```python
from build123d import *

# Parameters (mm, degrees)
SKETCH1_W           = 740
SKETCH1_H           = 720
SKETCH1_W_2         = 720
SKETCH1_H_2         = 700
BOSS_EXTRUDE1_DEPTH = 15
SKETCH2_R           = 2.5
CUT_EXTRUDE1_DEPTH  = 517.454257413
SKETCH3_W           = 20
SKETCH3_H           = 10
CUT_EXTRUDE2_DEPTH  = 20
SKETCH5_W           = 20
SKETCH5_H           = 10
CUT_EXTRUDE3_DEPTH  = 20
SKETCH6_W           = 20
SKETCH6_H           = 30
SKETCH6_W_2         = 30
SKETCH6_H_2         = 20
BOSS_EXTRUDE2_DEPTH = 4
SKETCH7_R           = 2
CUT_EXTRUDE4_DEPTH  = 4


with BuildPart() as part:
    # Sketch1 → Boss-Extrude1 (new body)
    with BuildSketch(Plane(origin=(0, 0, 0), x_dir=(1, 0, 0), z_dir=(0, 1, 0))):
        Rectangle(SKETCH1_W, SKETCH1_H)
        Rectangle(SKETCH1_W_2, SKETCH1_H_2, mode=Mode.SUBTRACT)
    extrude(amount=BOSS_EXTRUDE1_DEPTH)

    # Sketch2 → Cut-Extrude1 (cut, through all)
    with BuildSketch(Plane(origin=(0, 15, 0), x_dir=(1, 0, 0), z_dir=(0, 1, 0))):
        with Locations(Location((-365, 355, 0), (0, 0, 270))):
            Circle(SKETCH2_R)
        with Locations(Location((365, 355, 0), (0, 0, 270))):
            Circle(SKETCH2_R)
        with Locations(Location((365, -355, 0), (0, 0, 270))):
            Circle(SKETCH2_R)
        with Locations(Location((-365, -355, 0), (0, 0, 270))):
            Circle(SKETCH2_R)
    extrude(amount=-CUT_EXTRUDE1_DEPTH, mode=Mode.SUBTRACT)

    # Sketch3 → Cut-Extrude2 (cut)
    with BuildSketch(Plane.XY.offset(360)):
        with Locations((-360, 7.5)):
            Rectangle(SKETCH3_W, SKETCH3_H)
        with Locations((360, 7.5)):
            Rectangle(SKETCH3_W, SKETCH3_H)
    extrude(amount=-CUT_EXTRUDE2_DEPTH, mode=Mode.SUBTRACT)

    # Sketch5 → Cut-Extrude3 (cut)
    with BuildSketch(Plane(origin=(0, 0, -360), x_dir=(-1, 0, 0), z_dir=(0, 0, -1))):
        with Locations((-360, 7.5)):
            Rectangle(SKETCH5_W, SKETCH5_H)
        with Locations((360, 7.5)):
            Rectangle(SKETCH5_W, SKETCH5_H)
    extrude(amount=-CUT_EXTRUDE3_DEPTH, mode=Mode.SUBTRACT)

    # Sketch6 → Boss-Extrude2 (add)
    with BuildSketch(Plane(origin=(0, 15, 0), x_dir=(1, 0, 0), z_dir=(0, 1, 0))):
        with Locations((-30, 335)):
            Rectangle(SKETCH6_W, SKETCH6_H)
        with Locations((30, 335)):
            Rectangle(SKETCH6_W, SKETCH6_H)
        with Locations((30, -335)):
            Rectangle(SKETCH6_W, SKETCH6_H)
        with Locations((-30, -335)):
            Rectangle(SKETCH6_W, SKETCH6_H)
        with Locations((-345, -38)):
            Rectangle(SKETCH6_W_2, SKETCH6_H_2)
        with Locations((-345, 38)):
            Rectangle(SKETCH6_W_2, SKETCH6_H_2)
        with Locations((345, -38)):
            Rectangle(SKETCH6_W_2, SKETCH6_H_2)
        with Locations((345, 38)):
            Rectangle(SKETCH6_W_2, SKETCH6_H_2)
    extrude(amount=-BOSS_EXTRUDE2_DEPTH)

    # Sketch7 → Cut-Extrude4 (cut)
    with BuildSketch(Plane(origin=(0, 15, 0), x_dir=(1, 0, 0), z_dir=(0, 1, 0))):
        with Locations(Location((-30, 330, 0), (0, 0, 270))):
            Circle(SKETCH7_R)
        with Locations(Location((30, 330, 0), (0, 0, 90))):
            Circle(SKETCH7_R)
        with Locations(Location((30, -330, 0), (0, 0, 270))):
            Circle(SKETCH7_R)
        with Locations(Location((-30, -330, 0), (0, 0, 90))):
            Circle(SKETCH7_R)
        with Locations(Location((340, 38, 0), (0, 0, 270))):
            Circle(SKETCH7_R)
        with Locations(Location((340, -38, 0), (0, 0, 90))):
            Circle(SKETCH7_R)
        with Locations(Location((-340, -38, 0), (0, 0, 270))):
            Circle(SKETCH7_R)
        with Locations(Location((-340, 38, 0), (0, 0, 90))):
            Circle(SKETCH7_R)
    extrude(amount=-CUT_EXTRUDE4_DEPTH, mode=Mode.SUBTRACT)


solid = part.part
```
For this review, take the finished solid that the model builds, in its own axes (mm). A direction names the side the tool comes from. Give positions to 0.01 mm unless a question says otherwise; leave off trailing zeros. Write each loop counter-clockwise with the first axis right and the second up, starting at its lowest first coordinate (ties: lowest second). Pieces come first, ordered by that corner, then holes. Notation, with made-up numbers: M 21.5,53.5 L 49.5,53.5 A15 ccw 49.5,57.5 Z; hole C 67,52.5 d5. An arc over 180 degrees is marked long. One line per item, written item: value.
1) Take a section at C-C, the plane x = -73. Write out the cut boundary in (y, z).
Results are:
outline: M 0,-360 L 15,-360 L 15,-350 L 0,-350 Z; M 0,350 L 15,350 L 15,360 L 0,360 Z
2) For P1, Ø8, axis at x = 365, z = 355, coming from the +Y side; P2, Ø16, axis at x = 350.5, z = -40.5, coming from the -Y side; P3, Ø3, axis at y = 10, z = 355, coming from the +X side, all flat-tipped, find the tip position at first contact; note any pin that passes through.
Results are:
P1: stops at y = 15
P2: stops at y = 11
P3: stops at x = 350
3) For faces 3 (the flat face through (362, 2.5, 352)), 4 (the flat face through (362, 2.5, -352)), 5 (the flat face through (-345, 11, 38)), 6 (the flat face through (-362, 12.5, -352)), list the 3-axis set-ups (+Z, -Z, +X, -X, +Y, -Y) from which the entire face can be reached by the end or side of a thin tool; tool diameter is ignored.
Results are:
face 3: +Z, +X
face 4: -Z, +X
face 5: -Y
face 6: -Z, -X
4) For line 1 (Z direction, x = -340, y = 14.1); line 2 (X direction, y = 13.1, z = 38); line 3 (X direction, y = 1.6, z = -355), list the stretches that pass through material, from the lowest coordinate up. Write a range as from..to.
Results are:
line 1: z = -360..-350, -48..-40, -36..-28, 28..36, 40..48, 350..360
line 2: x = -370..-342, -338..-330, 330..338, 342..370
line 3: x = -370..-367.5, -362.5..362.5, 367.5..370
5) Take a section at B-B, the plane z = 101.5. Write out the cut boundary in (x, y), then the cut area to 3 significant figures.
Results are:
outline: M -370,0 L -360,0 L -360,15 L -370,15 Z; M 360,0 L 370,0 L 370,15 L 360,15 Z
area: 300 mm²
6) Take a section at A-A, the plane y = 5.5. Write out the cut boundary in (x, z).
Results are:
outline: M -370,-340 L -360,-340 L -360,340 L -370,340 Z; M -350,-360 L 350,-360 L 350,-350 L -350,-350 Z; M -350,350 L 350,350 L 350,360 L -350,360 Z; M 360,-340 L 370,-340 L 370,340 L 360,340 Z
7) The part is to be moulded in two halves that separate along X. For faces 1 (the flat face through (30, 11, 335)), 2 (the flat face through (362, 12.5, -352)), say which applies: +X half, -X half, draft (parallel to the pull), parting line (faces both ways), or undercut.
Results are:
face 1: undercut
face 2: draft
